```python
from build123d import *

# Parameters (mm, degrees)
F1_DEPTH = 3


with BuildPart() as f1:
    # F0 (on Front) → F1 (new body)
    with BuildSketch(Plane.XZ):
        with BuildLine():
            Line((75, 25), (75, 35))
            Line((75, 35), (68.875617, 35))
            ThreePointArc((68.875617, 35), (65.658037, 33.827163), (63.949936, 30.858872))
            Line((63.949936, 30.858872), (55.803943, -15.858872))
            ThreePointArc((55.803943, -15.858872), (54.095841, -18.827163), (50.878261, -20))
            Line((50.878261, -20), (0, -20))
            Line((0, -20), (-50.878261, -20))
            ThreePointArc((-50.878261, -20), (-54.095841, -18.827163), (-55.803943, -15.858872))
            Line((-55.803943, -15.858872), (-63.949936, 30.858872))
            ThreePointArc((-63.949936, 30.858872), (-65.658037, 33.827163), (-68.875617, 35))
            Line((-68.875617, 35), (-75, 35))
            Line((-75, 35), (-75, 25))
            Line((-75, 25), (-72, 25))
            Line((-72, 25), (-72, 15))
            Line((-72, 15), (-75, 15))
            Line((-75, 15), (-75, 5))
            Line((-75, 5), (-72, 5))
            Line((-72, 5), (-72, -5))
            Line((-72, -5), (-75, -5))
            Line((-75, -5), (-75, -15))
            Line((-75, -15), (-72, -15))
            Line((-72, -15), (-72, -25))
            Line((-72, -25), (-75, -25))
            Line((-75, -25), (-75, -32))
            Line((-75, -32), (-63.461538, -32))
            Line((-63.461538, -32), (-63.461538, -35))
            Line((-63.461538, -35), (-51.923077, -35))
            Line((-51.923077, -35), (-51.923077, -32))
            Line((-51.923077, -32), (-40.384615, -32))
            Line((-40.384615, -32), (-40.384615, -35))
            Line((-40.384615, -35), (-28.846154, -35))
            Line((-28.846154, -35), (-28.846154, -32))
            Line((-28.846154, -32), (-17.307692, -32))
            Line((-17.307692, -32), (-17.307692, -35))
            Line((-17.307692, -35), (-5.769231, -35))
            Line((-5.769231, -35), (-5.769231, -32))
            Line((-5.769231, -32), (5.769231, -32))
            Line((5.769231, -32), (5.769231, -35))
            Line((5.769231, -35), (17.307692, -35))
            Line((17.307692, -35), (17.307692, -32))
            Line((17.307692, -32), (28.846154, -32))
            Line((28.846154, -32), (28.846154, -35))
            Line((28.846154, -35), (40.384615, -35))
            Line((40.384615, -35), (40.384615, -32))
            Line((40.384615, -32), (51.923077, -32))
            Line((51.923077, -32), (51.923077, -35))
            Line((51.923077, -35), (63.461538, -35))
            Line((63.461538, -35), (63.461538, -32))
            Line((63.461538, -32), (75, -32))
            Line((75, -32), (75, -25))
            Line((75, -25), (72, -25))
            Line((72, -25), (72, -15))
            Line((72, -15), (75, -15))
            Line((75, -15), (75, -5))
            Line((75, -5), (72, -5))
            Line((72, -5), (72, 5))
            Line((72, 5), (75, 5))
            Line((75, 5), (75, 15))
            Line((75, 15), (72, 15))
            Line((72, 15), (72, 25))
            Line((72, 25), (75, 25))
        make_face()
    extrude(amount=F1_DEPTH)


solid = f1.part
```
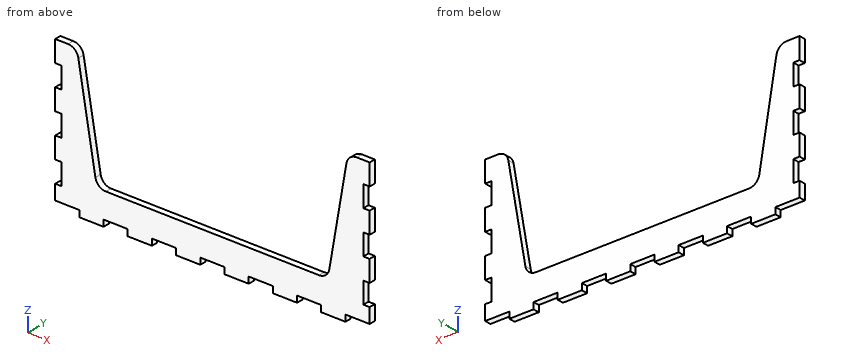
Can you work these out from the model? Positions are in its coordinate system, mm. Coordinates: 2 decimals unless noted, no trailing zeros. Loops run counter-clockwise (first coordinate to the right, second up) from the corner with the lowest first, then second, coordinate; pieces in that order, holes last.
1) I need wall thicknesses on probe 1 along X at (y, z) = (-2.7, 31); probe 2 along Z at (x, y) = (-30, -1.1); probe 3 along X at (y, z) = (-2.4, -20.5). Which ranges of each line are inside material? Lowest first, please.
2) Imagine slicing it at D-D on z = 10. List the corners of the cut face in (x, y) for me, plus the area to 3 significant figures.
3) Imagine slicing it at B-B on x = 3. List the corners of the cut face in (y, z) for me, plus the area to 3 significant figures.
4) Imagine slicing it at A-A on z = 1.5. List the corners of the cut face in (x, y) for me.
5) For pin 1 (0.9 mm diameter, centred on y = -1.5, z = -34, fed in from -X); pin 2 (1.5 mm diameter, centred on x = 73, y = -1, fed in from -Z); pin 3 (1 mm diameter, centred on x = 40, y = -2, fed in from +Z), each with a flat end and sliding along its axis, tell me the tip position at first contact or that it passes through.
6) Imagine slicing it at C-C on z = -23. List the corners of the cut face in (x, y) for me, plus the area to 3 significant figures.
Completed:
1. probe 1: x = -75 to -63.98, 63.98 to 75
1. probe 2: z = -35 to -20
1. probe 3: x = -72 to 72
2. outline: (-75, -3) - (-60.31, -3) - (-60.31, 0) - (-75, 0) - close; (60.31, -3) - (75, -3) - (75, 0) - (60.31, 0) - close
2. area: 88.1 mm2
3. outline: (-3, -32) - (0, -32) - (0, -20) - (-3, -20) - close
3. area: 36.0 mm2
4. outline: (-72, -3) - (-58.83, -3) - (-58.83, 0) - (-72, 0) - close; (58.83, -3) - (72, -3) - (72, 0) - (58.83, 0) - close
5. pin 1: stops at x = -63.46
5. pin 2: stops at z = -32
5. pin 3: stops at z = -20
6. outline: (-72, -3) - (72, -3) - (72, 0) - (-72, 0) - close
6. area: 432 mm2
